The listing builds one solid part. Answer for the finished solid, in the listing's coordinates (mm). Face numbers are marked on the shaded views. A direction names the side the tool comes from. Give positions to 0.01 mm unless a question says otherwise; leave off trailing zeros. Loops run counter-clockwise (first coordinate to the right, second up) from the corner with the lowest first, then second, coordinate; pieces in that order, holes last. Notation, with made-up numbers: M 14,-27.5 L 51,-27.5 A23 cw 51,0.5 Z; hole C -4.5,-25.5 d8. An arc over 180 degrees is marked long. One line per item, written item: value. Start each with the question number.
Q1. Consider L1, parallel to Y at x = 43.18, z = 8.75; L2, parallel to X at y = 17.5, z = 6.5; L3, parallel to X at y = 4, z = 12.75. Determine where each line is inside the solid, lowest interval first.
Q2. Flat-ended cylindrical pins translate along their axes: pin 1 (20.5 mm diameter, centred on x = 1, y = 12.5, fed in from +Z); pin 2 (10 mm diameter, centred on x = -29, y = -5, fed in from -Z); pin 3 (1.3 mm diameter, centred on y = 7, z = -1, fed in from +X). Find the tip coordinate at first contact, or state that the pin passes through.
Q3. For the marked faces 5, 6 and 7, determine the directions among +Z, -Z, +X, -X, +Y, -Y from which every point of the face is accessible in a straight line to the end or side of a thin tool.
Q4. The mould has two halves that part along X. Classify the marked faces 1, 2, 3 and 4: +X half, -X half, draft (parallel to the pull), parting line (faces both ways), or undercut.
Q5. A cutting plane is placed at C-C, the plane y = -6. Determine the outline of the cut face in (x, z), and give its area (3 significant figures).
Q6. A cutting plane is placed at B-B, the plane y = -17.78. Determine the outline of the cut face in (x, z).
Q7. A cutting plane is placed at A-A, the plane x = -43.18. Determine the outline of the cut face in (y, z), and give its area (3 significant figures).
Q8. A cutting plane is placed at D-D, the plane z = -1.25. Determine the outline of the cut face in (x, y), and give its area (3 significant figures).
from build123d import *

# Parameters (mm, degrees)
F0_W     = 38.1
F0_H     = 50.8
F0_W_2   = 25.4
F1_DEPTH = 12.7
F2_DEPTH = 15.24
F5_W     = 12.7
F5_H     = 2.54
F6_DEPTH = 50.8
F7_R     = 5.059721
F8_DEPTH = 17.781


with BuildPart() as f1:
    # F0 (on Top) → F1 (new body)
    with BuildSketch(Plane.XY):
        with Locations((-31.75, 0)):
            Rectangle(F0_W, F0_H)
        Rectangle(F0_W_2, F0_H)
        with Locations((31.75, 0)):
            Rectangle(F0_W, F0_H)
    extrude(amount=F1_DEPTH)

    # F0 (on Top) → F2 (join)
    with BuildSketch(Plane.XY):
        with Locations((31.75, 0)):
            Rectangle(F0_W, F0_H)
        with Locations((-31.75, 0)):
            Rectangle(F0_W, F0_H)
    extrude(amount=F2_DEPTH)

    # F5 (on face) → F6 (join)
    with BuildSketch(Plane.XZ.offset(25.4)):
        with Locations((-6.35, -1.27)):
            Rectangle(F5_W, F5_H)
        with Locations((6.35, -1.27)):
            Rectangle(F5_W, F5_H)
    extrude(amount=-F6_DEPTH)

    # F7 (on face) → F8 (cut, through all)
    with BuildSketch(Plane.XY.offset(15.24)):
        with BuildLine():
            ThreePointArc((43.18, 22.839721), (39.602237, 14.202237), (48.239721, 17.78))
            ThreePointArc((48.239721, 17.78), (46.757763, 21.357763), (43.18, 22.839721))
        make_face()
        with Locations((43.18, -17.78)):
            Circle(F7_R)
        with Locations((-43.18, 17.78)):
            Circle(F7_R)
        with Locations((-43.18, -17.78)):
            Circle(F7_R)
    extrude(amount=-F8_DEPTH, mode=Mode.SUBTRACT)


solid = f1.part
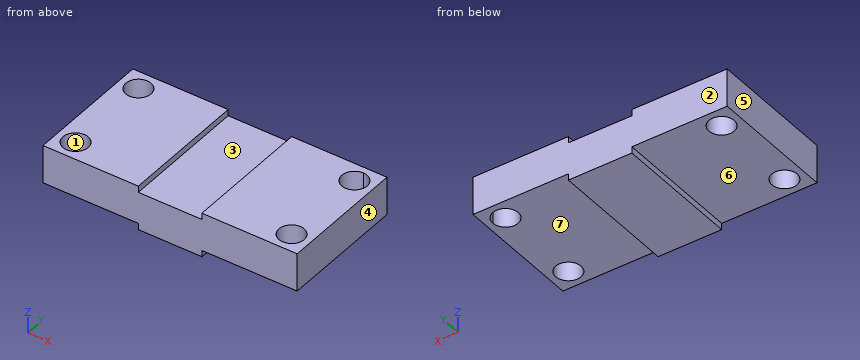
Answer block:
1. L1: -25.4 to -22.84, -12.72 to 12.72, 22.84 to 25.4
1. L2: -50.8 to -48.23, -38.13 to 38.13, 48.23 to 50.8
1. L3: -50.8 to -12.7, 12.7 to 50.8
2. pin 1: z = 12.7
2. pin 2: z = 0
2. pin 3: x = 12.7
3. face 5: +Z, -Z, -X, +Y, -Y
3. face 6: -Z, -X, +Y, -Y
3. face 7: -Z, +X, +Y, -Y
4. face 1: undercut
4. face 2: draft
4. face 3: undercut
4. face 4: +X half
5. outline: M -50.8,0 L -12.7,0 L -12.7,-2.54 L 12.7,-2.54 L 12.7,0 L 50.8,0 L 50.8,15.24 L 12.7,15.24 L 12.7,12.7 L -12.7,12.7 L -12.7,15.24 L -50.8,15.24 Z
5. area: 1,550 mm^2
6. outline: M -50.8,0 L -48.24,0 L -48.24,15.24 L -50.8,15.24 Z; M -38.12,0 L -12.7,0 L -12.7,-2.54 L 12.7,-2.54 L 12.7,0 L 38.12,0 L 38.12,15.24 L 12.7,15.24 L 12.7,12.7 L -12.7,12.7 L -12.7,15.24 L -38.12,15.24 Z; M 48.24,0 L 50.8,0 L 50.8,15.24 L 48.24,15.24 Z
7. outline: M -25.4,0 L -22.84,0 L -22.84,15.24 L -25.4,15.24 Z; M -12.72,0 L 12.72,0 L 12.72,15.24 L -12.72,15.24 Z; M 22.84,0 L 25.4,0 L 25.4,15.24 L 22.84,15.24 Z
7. area: 466 mm^2
8. outline: M -12.7,-25.4 L 12.7,-25.4 L 12.7,25.4 L -12.7,25.4 Z
8. area: 1,290 mm^2
